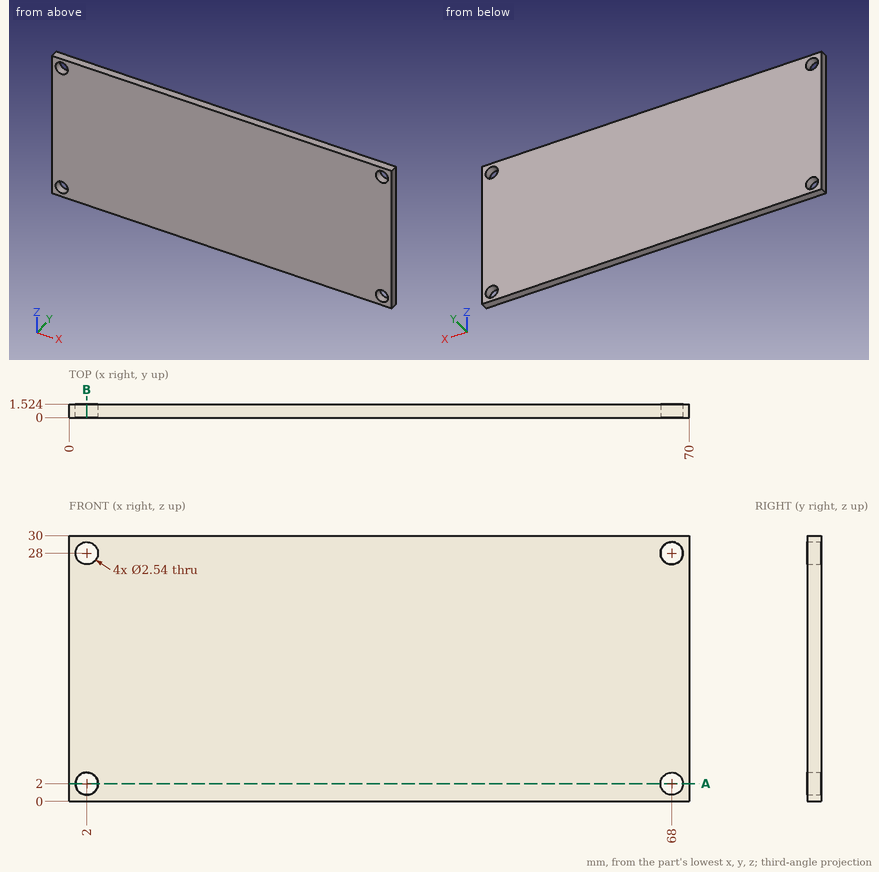
Here's the drawing with two shaded views (mm, measured from the low corner). I have some questions. Round coordinates to 2 decimals unless told otherwise and drop trailing zeros. Loops run counter-clockwise (first coordinate to the right, second up) from the corner with the lowest first, then second, coordinate; pieces in that order, holes last. Notation, with made-up numbers: M 31.5,36.25 L 51.5,36.25 A16 ccw 51.5,52.25 Z; hole C -24,-35 d8. An arc over 180 degrees is marked long. Answer as a JSON object with one key per item and string values. Group by question number.
Q1. Imagine slicing it at A-A, the plane z = 2. Please give me the cut outline in (x, y), then the cut area to 3 significant figures.
Q2. Will this pin go through, and if not, where does the flat tip stop? pin 1 (1.5 mm diameter, centred on x = 68, z = 28, fed in from +Y).
Q3. Imagine slicing it at B-B, the plane x = 2. Please give me the cut outline in (y, z), then the cut area to 3 significant figures.
Q4. Please list where these lines run through material, in increasing order: L1, parallel to X at y = 0.95, z = 28; L2, parallel to Z at x = 2, y = 0.55; L3, parallel to X at y = 1.15, z = 28.5.
Findings:
{
 "1": {"outline": "M 0,0 L 0.73,0 L 0.73,1.52 L 0,1.52 Z; M 3.27,0 L 66.73,0 L 66.73,1.52 L 3.27,1.52 Z; M 69.27,0 L 70,0 L 70,1.52 L 69.27,1.52 Z", "area": "98.9 mm2"},
 "2": {"pin 1": "passes through"},
 "3": {"outline": "M 0,0 L 1.52,0 L 1.52,0.73 L 0,0.73 Z; M 0,3.27 L 1.52,3.27 L 1.52,26.73 L 0,26.73 Z; M 0,29.27 L 1.52,29.27 L 1.52,30 L 0,30 Z", "area": "38.0 mm2"},
 "4": {"L1": "x = 0 to 0.73, 3.27 to 66.73, 69.27 to 70", "L2": "z = 0 to 0.73, 3.27 to 26.73, 29.27 to 30", "L3": "x = 0 to 0.83, 3.17 to 66.83, 69.17 to 70"}
}
